For this review, take the finished solid that the model builds, in its own axes (mm). A direction names the side the tool comes from. Give positions to 0.01 mm unless a question says otherwise; leave off trailing zeros. Write each loop counter-clockwise with the first axis right and the second up, starting at its lowest first coordinate (ties: lowest second). Pieces come first, ordered by that corner, then holes. Notation, with made-up numbers: (-25, 41) -> (-2, 41) arc R31 ccw to (-2, 71) -> close; hole circle Ø7 at (-18.5, 36.25). An arc over 180 degrees is marked (long way). Answer as CSV lines item,"result".
```python
from build123d import *

# Parameters (mm, degrees)
SKETCH_1_W          = 118
SKETCH_1_H          = 25.5
EXTRUDE_1_DEPTH     = 75.5
SKETCH_2_W          = 6
SKETCH_2_H          = 17.25
CUT_EXTRUDE_1_DEPTH = 72.5
CUT_EXTRUDE_2_DEPTH = 141.820808122
SKETCH_4_R          = 2
CUT_EXTRUDE_3_DEPTH = 142.144650979


with BuildPart() as part:
    # 草图1 → 凸台-拉伸1 (new body)
    with BuildSketch(Plane(origin=(0, 0, 0), x_dir=(1, 0, 0), z_dir=(0, 1, 0))):
        with Locations((59, -12.75)):
            Rectangle(SKETCH_1_W, SKETCH_1_H)
    extrude(amount=EXTRUDE_1_DEPTH)

    # 草图2 → 切除-拉伸1 (cut)
    with BuildSketch(Plane(origin=(0, 75.5, 0), x_dir=(1, 0, 0), z_dir=(0, 1, 0))):
        with Locations((3, -8.625)):
            Rectangle(SKETCH_2_W, SKETCH_2_H)
        with Locations((115, -8.625)):
            Rectangle(SKETCH_2_W, SKETCH_2_H)
    extrude(amount=-CUT_EXTRUDE_1_DEPTH, mode=Mode.SUBTRACT)

    # 草图3 → 切除-拉伸2 (cut, through all)
    with BuildSketch(Plane(origin=(0, 3, 0), x_dir=(1, 0, 0), z_dir=(0, 1, 0))):
        with BuildLine():
            Line((0, -13.75), (3, -13.75))
            ThreePointArc((3, -13.75), (5.25, -11.5), (3, -9.25))
            Line((3, -9.25), (0, -9.25))
            Line((0, -9.25), (0, -13.75))
        make_face()
        with BuildLine():
            Line((118, -13.75), (118, -9.25))
            Line((118, -9.25), (115, -9.25))
            ThreePointArc((115, -9.25), (112.75, -11.5), (115, -13.75))
            Line((115, -13.75), (118, -13.75))
        make_face()
    extrude(amount=-CUT_EXTRUDE_2_DEPTH, mode=Mode.SUBTRACT)

    # 草图4 → 切除-拉伸3 (cut, through all)
    with BuildSketch(Plane(origin=(0, 0, 17.25), x_dir=(-1, 0, 0), z_dir=(0, 0, -1))):
        with Locations((-115, 50.2)):
            Circle(SKETCH_4_R)
        with Locations((-115, 27.7)):
            Circle(SKETCH_4_R)
        with Locations((-3, 50.2)):
            Circle(SKETCH_4_R)
        with Locations((-3, 27.7)):
            Circle(SKETCH_4_R)
    extrude(amount=-CUT_EXTRUDE_3_DEPTH, mode=Mode.SUBTRACT)


solid = part.part
```
Q1. Add section B-B (z = 3.75). Write out the cut boundary in (x, y), plus the area to 3 significant figures.
Answer block:
outline,"(0, 0) -> (118, 0) -> (118, 3) -> (112, 3) -> (112, 75.5) -> (6, 75.5) -> (6, 3) -> (0, 3) -> close"
area,"8,040 mm2"
Q2. Add section A-A (y = 27.7). Write out the cut boundary in (x, z), plus the area to 3 significant figures.
Answer block:
outline,"(0, 17.25) -> (1, 17.25) -> (1, 25.5) -> (0, 25.5) -> close; (5, 17.25) -> (6, 17.25) -> (6, 0) -> (112, 0) -> (112, 17.25) -> (113, 17.25) -> (113, 25.5) -> (5, 25.5) -> close; (117, 17.25) -> (118, 17.25) -> (118, 25.5) -> (117, 25.5) -> close"
area,"2,740 mm2"
Q3. For faces 1 (the flat face through (2, 2, 9.25)), 2 (the flat face through (58, 0, 13)), 3 (the flat face through (115, 40, 17.25)), 4 (the cylindrical face through (2.077, 48.426, 21.317)), 5 (the flat face through (3, 40, 17.25)), list the 3-axis set-ups (+Z, -Z, +X, -X, +Y, -Y) from which the entire face can be reached by the end or side of a thin tool; tool diameter is ignored.
Answer block:
face 1,"-X, +Y, -Y"
face 2,"+Z, -Z, +X, -X, -Y"
face 3,"-Z, +X, +Y"
face 4,"+Z, -Z"
face 5,"-Z, -X, +Y"
Q4. To check wall thickness, follow probe 1 along Y at (x, z) = (115, 22); probe 2 along X at (y, z) = (44.5, 16.25). State the ranges of each line that lie inside material, in increasing order. Write a range as [from, to].
Answer block:
probe 1,"y = [0, 25.7], [29.7, 48.2], [52.2, 75.5]"
probe 2,"x = [6, 112]"
Q5. Clearance check with flat-ended pins moving along their axes: pin 1 (2 mm diameter, centred on y = 60, z = 5, fed in from +X); pin 2 (3 mm diameter, centred on x = 115, y = 50.2, fed in from +Z); pin 3 (8.5 mm diameter, centred on y = 42.5, z = 8, fed in from -X); pin 4 (3 mm diameter, centred on x = 2.5, z = 9.5, fed in from +Y). State where each tip first meets the part, or that it passes through.
Answer block:
pin 1,"stops at x = 112"
pin 2,"passes through"
pin 3,"stops at x = 6"
pin 4,"stops at y = 3"
Q6. Add section C-C (y = 14.5). Write out the cut boundary in (x, z), plus the area to 3 significant figures.
Answer block:
outline,"(0, 17.25) -> (6, 17.25) -> (6, 0) -> (112, 0) -> (112, 17.25) -> (118, 17.25) -> (118, 25.5) -> (0, 25.5) -> close"
area,"2,800 mm2"
Q7. Draft analysis for pull direction Z (two halves, no side actions). For faces 6 (the flat face through (117, 2, 9.25)), 7 (the flat face through (58, 37, 0)), 8 (the cylindrical face through (116.998, 50.288, 21.317)), 9 (the cylindrical face through (112.75, 1.52, 11.45)), state which applies: released by +Z, released by -Z, zero draft, split by the parting line, or undercut.
Answer block:
face 6,"undercut"
face 7,"released by -Z"
face 8,"zero draft"
face 9,"undercut"
